Can you work these out from the drawing? Everything is in mm from the part's minimum corner. A direction names the side the tool comes from. Coordinates: 2 decimals unless noted, no trailing zeros. Write each loop counter-clockwise with the first axis right and the second up, starting at its lowest first coordinate (ties: lowest second). Pieces come first, ordered by that corner, then holes. Notation, with made-up numbers: M 50.5,34 L 59.5,34 A19 ccw 59.5,48 Z; hole C -12.75,89.5 d4. An arc over 180 degrees is marked long. Answer as a JSON object with one key per item and string values. Group by question number.
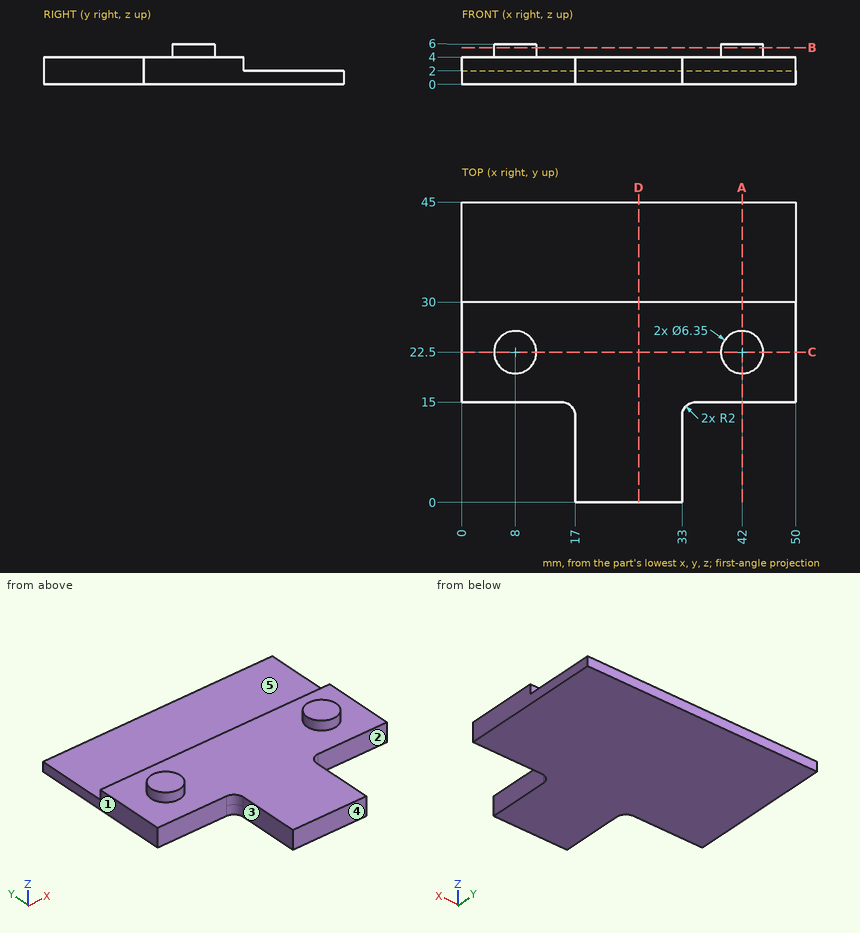
Q1. Please list where these lines run through material, in increasing order: L1, parallel to Z at x = 40, y = 25; L2, parallel to Z at x = 35, y = 42; L3, parallel to Y at x = 12.5, z = 3.1.
Q2. If we section it at A-A on x = 42: List the corners of the cut face in (y, z) for me (3 decimals).
Q3. On a 3-axis mill with a long thin cutter (end or side, diameter ignored), from which of +Z, -Z, +X, -X, +Y, -Y can I reach the whole of each face in a straight line? I mean the marked faces 1, 2, 3, 4 and 5. Say none if no direction works.
Q4. If we section it at C-C on y = 22.5: List the corners of the cut face in (x, z) for me (3 decimals).
Q5. If we section it at B-B on z = 5.45: List the corners of the cut face in (x, y) for me (3 decimals).
Q6. If we section it at D-D on x = 26.5: List the corners of the cut face in (y, z) for me, and give its area (3 significant figures).
Q7. Will these pins go through, and if not, where does the flat tip stop? pin 1 (0.6 mm diameter, centred on x = 29, z = 3, fed in from +Y); pin 2 (2 mm diameter, centred on x = 41.5, z = 1.5, fed in from -Y); pin 3 (5 mm diameter, centred on x = 14.5, y = 18, fed in from +Z).
Reply:
{
 "1": {"L1": "0 to 4", "L2": "0 to 2", "L3": "15 to 30"},
 "2": {"outline": "M 15,0 L 45,0 L 45,2 L 30,2 L 30,4 L 25.675,4 L 25.675,6 L 19.325,6 L 19.325,4 L 15,4 Z"},
 "3": {"face 1": "+Z, -Z, -X, +Y, -Y", "face 2": "+Z, -Z, +X, -Y", "face 3": "+Z, -Z, -X, -Y", "face 4": "+Z, -Z, +X, -X, -Y", "face 5": "+Z, +X, -X, +Y"},
 "4": {"outline": "M 0,0 L 50,0 L 50,4 L 45.175,4 L 45.175,6 L 38.825,6 L 38.825,4 L 11.175,4 L 11.175,6 L 4.825,6 L 4.825,4 L 0,4 Z"},
 "5": {"outline": "C 8,22.5 d6.35; C 42,22.5 d6.35"},
 "6": {"outline": "M 0,0 L 45,0 L 45,2 L 30,2 L 30,4 L 0,4 Z", "area": "150 mm^2"},
 "7": {"pin 1": "y = 30", "pin 2": "y = 15", "pin 3": "z = 4"}
}
